Part print with two shaded views. Sizes in mm from the minimum x, y, z corner. A direction names the side the tool comes from. Coordinates: 2 decimals unless noted, no trailing zeros. Loops run counter-clockwise (first coordinate to the right, second up) from the corner with the lowest first, then second, coordinate; pieces in that order, holes last.
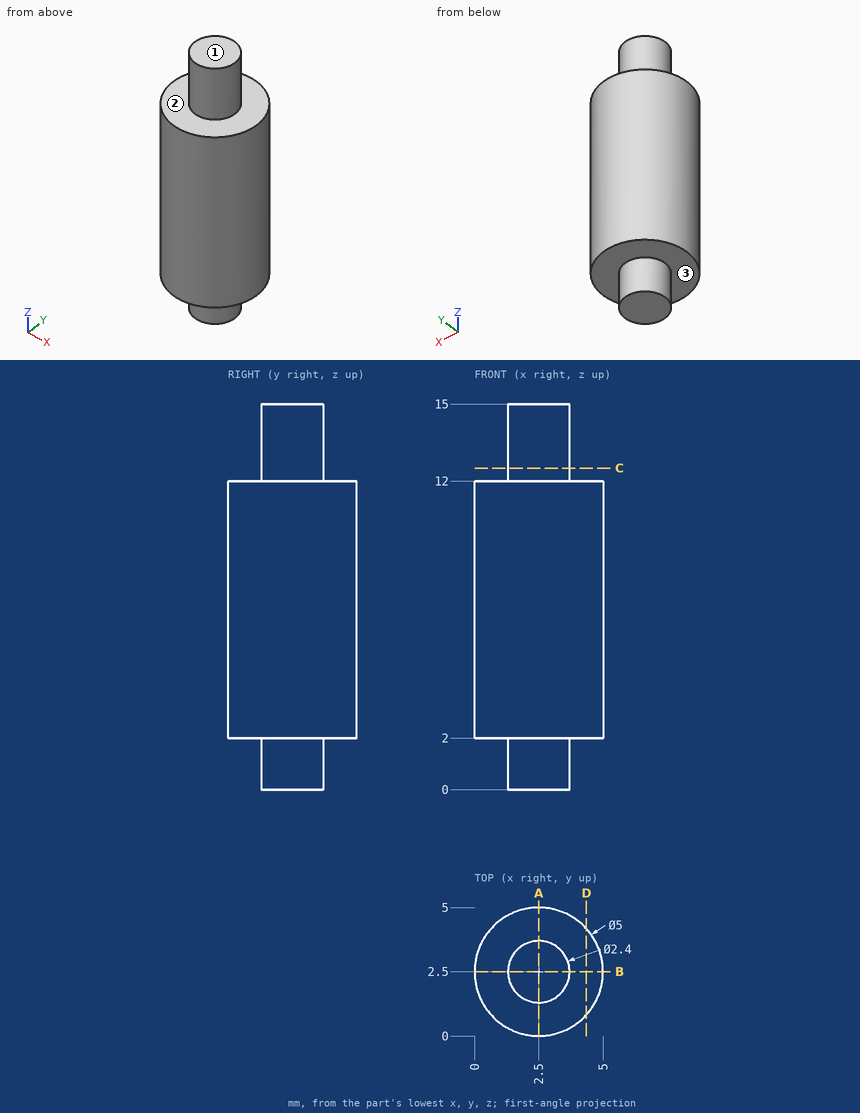
Q1. Which spindle directions (+Z, -Z, +X, -X, +Y, -Y) get a long thin tool onto all of the face, cutting with end or side? Do the marked faces 1, 2 and 3. Say none if no direction does.
Answers:
face 1: +Z, +X, -X, +Y, -Y
face 2: +Z
face 3: -Z
Q2. Flat gauge pins, fed straight in: P1, Ø1.5, axis at x = 1.5, z = 7, coming from the +Y side; P2, Ø1.5, axis at y = 3.5, z = 8.5, coming from the -X side; P3, Ø1.5, axis at x = 1.5, y = 4, coming from the +Z side; P4, Ø2, axis at y = 1, z = 6.5, coming from the -X side. Where does each tip first touch, or does it go through?
Answers:
P1: stops at y = 4.99
P2: stops at x = 0.01
P3: stops at z = 15
P4: stops at x = 0.05
Q3. Slice it at C-C (z = 12.5). List the corners of the cut face in (x, y), and give its area (3 significant figures).
Answers:
outline: circle Ø2.4 at (2.5, 2.5)
area: 4.52 mm2
Q4. Slice it at D-D (x = 4.35). List the corners of the cut face in (y, z), and give its area (3 significant figures).
Answers:
outline: (0.82, 2) - (4.18, 2) - (4.18, 12) - (0.82, 12) - close
area: 33.6 mm2
Q5. Drill centre lines: line 1 (Z direction, x = 0.3, y = 2); line 2 (Y direction, x = 2.4, z = 13.5); line 3 (Y direction, x = 3, z = 9.5). Where is each one in solid material? Low to high.
Answers:
line 1: z = 2 to 12
line 2: y = 1.3 to 3.7
line 3: y = 0.05 to 4.95
Q6. Slice it at A-A (x = 2.5). List the corners of the cut face in (y, z), and give its area (3 significant figures).
Answers:
outline: (0, 2) - (1.3, 2) - (1.3, 0) - (3.7, 0) - (3.7, 2) - (5, 2) - (5, 12) - (3.7, 12) - (3.7, 15) - (1.3, 15) - (1.3, 12) - (0, 12) - close
area: 62.0 mm2
